```python
from build123d import *

# Parameters (mm, degrees)
F0_W     = 20
F0_H     = 15.5
F1_DEPTH = 5
F2_R     = 2.5
F3_DEPTH = 25
F4_DEPTH = 25


with BuildPart() as f1:
    # F0 (on Front) → F1 (new body)
    with BuildSketch(Plane.XZ):
        Rectangle(F0_W, F0_H)
    extrude(amount=F1_DEPTH)

    # F2 (on face) → F3 (cut)
    with BuildSketch(Plane.XZ.offset(5)):
        with Locations((-6, 0.25)):
            Circle(F2_R)
    extrude(amount=-F3_DEPTH, mode=Mode.SUBTRACT)

    # F2 (on face) → F4 (cut)
    with BuildSketch(Plane.XZ.offset(5)):
        with Locations((3.5, -0.75)):
            Circle(F2_R)
    extrude(amount=-F4_DEPTH, mode=Mode.SUBTRACT)


solid = f1.part
```
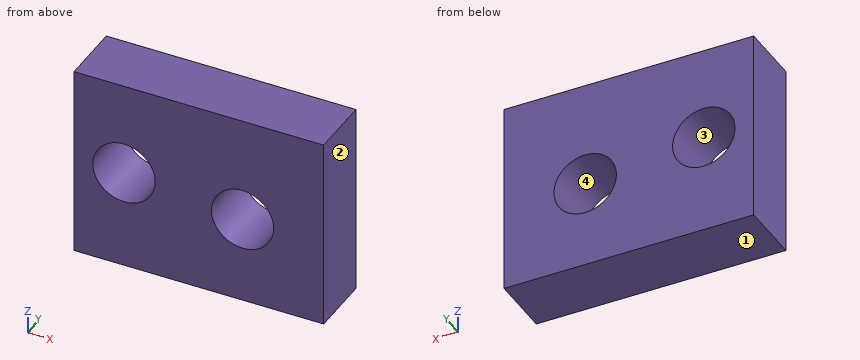
Model file for the job. Use its own axes, mm. Face numbers are marked on the shaded views. Round coordinates to 2 decimals unless told otherwise and drop trailing zeros. Order: outer loops, then holes, each group sorted by start corner. A loop starts at its lowest first (then second) coordinate and runs counter-clockwise, first axis right, second up. Notation, with made-up numbers: M 59,12.5 L 82,12.5 A13 ccw 82,20.5 Z; hole C -13,86 d11. An arc over 180 degrees is marked long. Use CSV: the item, a comma, the result in double quotes.
Item 1: Saw through at B-B (z = 2.5). List the corners of the cut face in (x, y), plus the area to 3 significant figures.
Worked answers:
outline,"M -10,-5 L -7.09,-5 L -7.09,0 L -10,0 Z; M -4.91,-5 L 10,-5 L 10,0 L -4.91,0 Z"
area,"89.1 mm²"
Item 2: Pull direction X, two halves, no side cores. Call the marked faces 1, 2, 3 and 4: released by +X, released by -X, zero draft, split by the parting line, or undercut.
Worked answers:
face 1,"zero draft"
face 2,"released by +X"
face 3,"undercut"
face 4,"undercut"
Item 3: Saw through at D-D (x = -7.75). List the corners of the cut face in (y, z).
Worked answers:
outline,"M -5,-7.75 L 0,-7.75 L 0,-1.54 L -5,-1.54 Z; M -5,2.04 L 0,2.04 L 0,7.75 L -5,7.75 Z"
Item 4: Probe probe 1 along Z at (x, y) = (-6, -1.3); probe 2 along X at (y, z) = (-0.85, 1.25); probe 3 along Z at (x, y) = (3, -4.3). List the from-to ranges inside material, lowest first.
Worked answers:
probe 1,"-7.75 to -2.25, 2.75 to 7.75"
probe 2,"-10 to -8.29, -3.71 to 2, 5 to 10"
probe 3,"-7.75 to -3.2, 1.7 to 7.75"
Item 5: Saw through at C-C (y = -2.55). List the corners of the cut face in (x, z), plus the area to 3 significant figures.
Worked answers:
outline,"M -10,-7.75 L 10,-7.75 L 10,7.75 L -10,7.75 Z; hole C -6,0.25 d5; hole C 3.5,-0.75 d5"
area,"271 mm²"
Item 6: Pin check, flat tip, straight feed: pin 1 (4.5 mm diameter, centred on x = -6, z = 0.25, fed in from -Y). Stop position of the tip, or through.
Worked answers:
pin 1,"through"
Item 7: Saw through at A-A (z = -0.25). List the corners of the cut face in (x, y).
Worked answers:
outline,"M -10,-5 L -8.45,-5 L -8.45,0 L -10,0 Z; M -3.55,-5 L 1.05,-5 L 1.05,0 L -3.55,0 Z; M 5.95,-5 L 10,-5 L 10,0 L 5.95,0 Z"
